The listing builds one solid part. Answer for the finished solid, in the listing's coordinates (mm). A direction names the side the tool comes from. Coordinates: 2 decimals unless noted, no trailing zeros. Loops run counter-clockwise (first coordinate to the right, second up) from the corner with the lowest first, then second, coordinate; pieces in that order, holes last. Notation, with made-up numbers: (12.5, 69.25) - (36.5, 69.25) arc R16 cw to (36.5, 82.25) - close; hole circle Ø9 at (-16.5, -30.5). An arc over 180 degrees is marked (long way). Put each result on its own line as item: value.
```python
from build123d import *

# Parameters (mm, degrees)
SKETCH1_W           = 12
SKETCH1_H           = 6.5
BOSS_EXTRUDE1_DEPTH = 10
SKETCH2_W           = 16
SKETCH2_H           = 10.5
BOSS_EXTRUDE2_DEPTH = 3
SKETCH3_W           = 12
SKETCH3_H           = 6.5
BOSS_EXTRUDE3_DEPTH = 25
BOSS_EXTRUDE4_DEPTH = 12
FILLET1_R           = 1
CUT_EXTRUDE1_REACH  = 41.186
SKETCH5_W           = 6
SKETCH5_H           = 0.672191444


with BuildPart() as part:
    # Sketch1 → Boss-Extrude1 (new body)
    with BuildSketch(Plane.XY):
        Rectangle(SKETCH1_W, SKETCH1_H)
    extrude(amount=BOSS_EXTRUDE1_DEPTH)

    # Sketch2 → Boss-Extrude2 (add)
    with BuildSketch(Plane.XY.offset(10)):
        Rectangle(SKETCH2_W, SKETCH2_H)
    extrude(amount=BOSS_EXTRUDE2_DEPTH)

    # Sketch3 → Boss-Extrude3 (add)
    with BuildSketch(Plane.XY.offset(13)):
        Rectangle(SKETCH3_W, SKETCH3_H)
    extrude(amount=BOSS_EXTRUDE3_DEPTH)

    # Sketch4 → Boss-Extrude4 (add)
    with BuildSketch(Plane(origin=(6, 0, 0), x_dir=(0, 0, -1), z_dir=(1, 0, 0))):
        Polygon((-10, 3.25), (0, 4), (0, 3.25), align=None)
        Polygon((-10, -3.25), (0, -4), (0, -3.25), align=None)
    extrude(amount=-BOSS_EXTRUDE4_DEPTH)

    # Fillet1
    fillet1_edges = [part.edges().sort_by_distance(p)[0] for p in [
        (0, -4, 0),
        (0, 4, 0),
    ]]
    fillet(fillet1_edges, radius=FILLET1_R)

    # Sketch5 → Cut-Extrude1 (cut, up to next)
    with BuildSketch(Plane(origin=(0, 0, 0), x_dir=(-1, 0, 0), z_dir=(0, 0, -1)), mode=Mode.PRIVATE) as cut_extrude1_sk1:
        with Locations((0, 3.586095722)):
            Rectangle(SKETCH5_W, SKETCH5_H)
    cut_extrude1_tool1 = extrude(cut_extrude1_sk1.sketch, amount=-CUT_EXTRUDE1_REACH, mode=Mode.PRIVATE) & part.part
    # Sketch5 → Cut-Extrude1 (cut, up to next)
    with BuildSketch(Plane(origin=(0, 0, 0), x_dir=(-1, 0, 0), z_dir=(0, 0, -1)), mode=Mode.PRIVATE) as cut_extrude1_sk2:
        with Locations((0, -3.586095722)):
            Rectangle(SKETCH5_W, SKETCH5_H)
    cut_extrude1_tool2 = extrude(cut_extrude1_sk2.sketch, amount=-CUT_EXTRUDE1_REACH, mode=Mode.PRIVATE) & part.part
    add(cut_extrude1_tool1.solids().sort_by_distance((0, 3.586096, 0))[0], mode=Mode.SUBTRACT)
    add(cut_extrude1_tool2.solids().sort_by_distance((0, -3.586096, 0))[0], mode=Mode.SUBTRACT)


solid = part.part
```
1) The part is cut by section C-C (z = 5). Give the vertices of the cut face in (x, y) (3 decimals).
Found:
outline: (-6, -3.625) - (-3, -3.625) - (-3, -3.25) - (3, -3.25) - (3, -3.625) - (6, -3.625) - (6, 3.625) - (3, 3.625) - (3, 3.25) - (-3, 3.25) - (-3, 3.625) - (-6, 3.625) - close
2) Each of these flat-tipped pins is pushed along its axis until it touches: pin 1 (0.7 mm diameter, centred on y = -3.5, z = 3, fed in from -X); pin 2 (2 mm diameter, centred on x = 4, z = 19.5, fed in from -Y); pin 3 (8 mm diameter, centred on x = 4, z = 30, fed in from +Y). Where does it stop, or does it pass through?
Found:
pin 1: stops at x = -6
pin 2: stops at y = -3.25
pin 3: stops at y = 3.25
3) For a pull along Z with two mould halves and no side action, classify faces 6 (the face through (-4.48, 3.58, 5.6)), 7 (the face through (4.52, 3.58, 5.6)), 8 (the face through (0, 0, 38)), 9 (the face through (0, -5.25, 11)) as pulls with the +Z half, pulls with the -Z half, needs draft (parallel to the pull), parting line crosses it, or undercut.
Found:
face 6: undercut
face 7: undercut
face 8: pulls with the +Z half
face 9: needs draft
4) The part is cut by section D-D (z = 16). Give the vertices of the cut face in (x, y), and give its area (3 significant figures).
Found:
outline: (-6, -3.25) - (6, -3.25) - (6, 3.25) - (-6, 3.25) - close
area: 78.0 mm^2
5) Straight lines are drawn through the part: L1, parallel to X at y = -1.75, z = 28; L2, parallel to Y at x = -2.5, z = 25.5; L3, parallel to Z at x = -7, y = -1. For each, find the intervals that lie inside material, in ascending order. Write a range as [from, to].
Found:
L1: x = [-6, 6]
L2: y = [-3.25, 3.25]
L3: z = [10, 13]
6) The part is cut by section A-A (x = 0.25). Give the vertices of the cut face in (y, z), and give its area (3 significant figures).
Found:
outline: (-5.25, 10) - (-3.25, 10) - (-3.25, 0.06) arc R1 ccw to (-2.92, 0) - (2.92, 0) arc R1 ccw to (3.25, 0.06) - (3.25, 10) - (5.25, 10) - (5.25, 13) - (3.25, 13) - (3.25, 38) - (-3.25, 38) - (-3.25, 13) - (-5.25, 13) - close
area: 259 mm^2
7) For faces 1 (the face through (0, -3.25, 5)), 2 (the face through (0, 3.25, 25)), 3 (the face through (6, 0, 25)), 4 (the face through (0, 3.25, 5)), 5 (the face through (0, -3.25, 25)), determine the directions among +Z, -Z, +X, -X, +Y, -Y from which every point of the face is accessible in a straight line to the end or side of a thin tool.
Found:
face 1: -Z, -Y
face 2: +Z, +X, -X, +Y
face 3: +Z, +X, +Y, -Y
face 4: -Z, +Y
face 5: +Z, +X, -X, -Y
8) The part is cut by section B-B (y = -2). Give the vertices of the cut face in (x, z).
Found:
outline: (-8, 10) - (-6, 10) - (-6, 0) - (6, 0) - (6, 10) - (8, 10) - (8, 13) - (6, 13) - (6, 38) - (-6, 38) - (-6, 13) - (-8, 13) - close
